Check sheet for the modelled part. Datum: model origin and axes. Units: mm. Face numbers are marked on the shaded views. A direction names the side the tool comes from. Coordinates: 2 decimals unless noted, no trailing zeros. Loops run counter-clockwise (first coordinate to the right, second up) from the corner with the lowest first, then second, coordinate; pieces in that order, holes last. Notation, with made-up numbers: M 24.25,70.25 L 48.25,70.25 A5 ccw 48.25,78.25 Z; hole C -28.75,-37 d11. An arc over 180 degrees is marked long. Use CSV: the item, a comma, the result in double quotes. Start each with the question number.
(1) Section check A-A on z = 0. Give the number of separate pieces and of enclosed holes in the cut face, and give its area (3 significant figures).
(2) Set-up check for the marked faces 1 and 2: record each of +Z, -Z, +X, -X, +Y, -Y from which the full face is reachable in a straight line by a thin tool's end or side.
(3) Section check B-B on y = 6. Record the cut outline in (x, z), and give its area (3 significant figures).
(4) Scan lines: line 1 (Y direction, x = 0.6, z = 0) (3 decimals); line 2 (Z direction, x = 0, y = 4); line 3 (Y direction, x = 0.25, z = 0.35). Record each from-to range of solid material in increasing order.
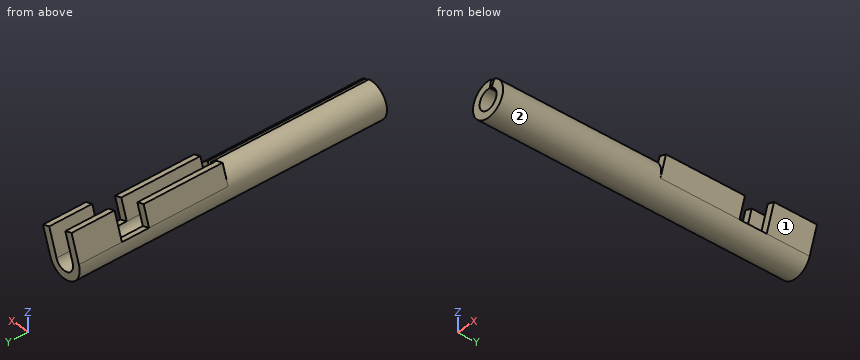
from build123d import *

# Parameters (mm, degrees)
EXTRUDE_THIN1_DEPTH = 6.35
EXTRUDE_THIN2_DEPTH = 3.175
EXTRUDE_THIN3_DEPTH = 1.0922
EXTRUDE_THIN4_DEPTH = 1.7272


with BuildPart() as part:
    # Sketch1 → Extrude-Thin1 (new body)
    with BuildSketch(Plane(origin=(0, 0, 0), x_dir=(1, 0, 0), z_dir=(0, 1, 0))):
        with BuildLine():
            ThreePointArc((0.288556611, -0.636111101), (-0.217707256, 0.66370611), (0.144278305, -0.683436918))
            Line((0.144278305, -0.683436918), (0.081320499, -0.385209899))
            ThreePointArc((0.081320499, -0.385209899), (-0.122707726, 0.374088898), (0.162640999, -0.358535348))
            Line((0.162640999, -0.358535348), (0.288556611, -0.636111101))
        make_face()
    extrude(amount=EXTRUDE_THIN1_DEPTH)

    # Sketch2 → Extrude-Thin2 (add)
    with BuildSketch(Plane(origin=(0, 6.35, 0), x_dir=(1, 0, 0), z_dir=(0, 1, 0))):
        with BuildLine():
            Line((0.916497603, -0.541281881), (0.662710919, 0.220718119))
            ThreePointArc((0.662710919, 0.220718119), (-0.220718119, 0.662710919), (-0.662710919, -0.220718119))
            Line((-0.662710919, -0.220718119), (-0.408924235, -0.982718119))
            Line((-0.408924235, -0.982718119), (-0.119741288, -0.886404758))
            Line((-0.119741288, -0.886404758), (-0.373527972, -0.124404758))
            ThreePointArc((-0.373527972, -0.124404758), (-0.124404758, 0.373527972), (0.373527972, 0.124404758))
            Line((0.373527972, 0.124404758), (0.627314657, -0.637595242))
            Line((0.627314657, -0.637595242), (0.916497603, -0.541281881))
        make_face()
    extrude(amount=EXTRUDE_THIN2_DEPTH)

    # Sketch3 → Extrude-Thin3 (add)
    with BuildSketch(Plane(origin=(0, 9.525, 0), x_dir=(1, 0, 0), z_dir=(0, 1, 0))):
        with BuildLine():
            ThreePointArc((0.662710919, 0.220718119), (-0.220718119, 0.662710919), (-0.662710919, -0.220718119))
            Line((-0.662710919, -0.220718119), (-0.373527972, -0.124404758))
            ThreePointArc((-0.373527972, -0.124404758), (-0.124404758, 0.373527972), (0.373527972, 0.124404758))
            Line((0.373527972, 0.124404758), (0.662710919, 0.220718119))
        make_face()
    extrude(amount=EXTRUDE_THIN3_DEPTH)

    # Sketch4 → Extrude-Thin4 (add)
    with BuildSketch(Plane(origin=(0, 10.6172, 0), x_dir=(1, 0, 0), z_dir=(0, 1, 0))):
        with BuildLine():
            Line((1.001093165, -0.795281881), (0.662710919, 0.220718119))
            ThreePointArc((0.662710919, 0.220718119), (-0.220718119, 0.662710919), (-0.662710919, -0.220718119))
            Line((-0.662710919, -0.220718119), (-0.324328673, -1.236718119))
            Line((-0.324328673, -1.236718119), (-0.035145727, -1.140404758))
            Line((-0.035145727, -1.140404758), (-0.373527972, -0.124404758))
            ThreePointArc((-0.373527972, -0.124404758), (-0.124404758, 0.373527972), (0.373527972, 0.124404758))
            Line((0.373527972, 0.124404758), (0.711910218, -0.891595242))
            Line((0.711910218, -0.891595242), (1.001093165, -0.795281881))
        make_face()
    extrude(amount=EXTRUDE_THIN4_DEPTH)


solid = part.part
Outcome:
1,separate pieces,"3"
1,enclosed holes,"0"
1,area,"7.27 mm²"
2,face 1,"-Z, +X, +Y, -Y"
2,face 2,"-Y"
3,outline,"M 0.08,0.39 L 0.14,0.68 A0.7 ccw long 0.29,0.64 L 0.16,0.36 A0.39 cw long Z"
3,area,"1.01 mm²"
4,line 1,"y = 0 to 9.525, 10.617 to 12.344"
4,line 2,"z = -0.7 to -0.39, 0.39 to 0.7"
4,line 3,"y = 0 to 6.35"
